Input: part model. Units: mm. Frame: model coordinates. A direction names the side the tool comes from. Round coordinates to 2 decimals unless told otherwise and drop trailing zeros. Write each loop counter-clockwise with the first axis right and the second up, starting at its lowest first coordinate (ties: lowest second). Pieces come first, ordered by that corner, then holes. Notation, with made-up numbers: (52.25, -31) -> (105.25, -31) arc R17 ccw to (105.25, -22) -> close; hole circle Ø2 at (55.25, 13.25). An arc over 180 degrees is marked (long way). Use CSV: the item, a comma, the result in double quotes.
Autodesk Inventor part; units mm, degrees
ref_plane "YZ Plane" through (0, 0, 0) normal (1, 0, 0) x (0, 1, 0)
ref_plane "XZ Plane" through (0, 0, 0) normal (0, 1, 0) x (-1, 0, 0)
ref_plane "XY Plane" through (0, 0, 0) normal (0, 0, 1) x (1, 0, 0)
sketch "Boceto1" plane through (0, 0, 0) normal (1, 0, 0) x (0, 1, 0)
  circle A0 centre (3, -6.5) radius 6.25
  line L0 (-9, 17.5) -> (-9, 20.5)
  line L1 (-9, 20.5) -> (3, 20.5)
  line L2 (3, 20.5) -> (3, 17.5)
  line L3 (3, 17.5) -> (40, 17.5)
  line L4 (40, 17.5) -> (40, -17.5)
  line L5 (40, -17.5) -> (3, -17.5)
  line L6 (3, -17.5) -> (3, -20.5)
  line L7 (3, -20.5) -> (-9, -20.5)
  line L8 (-9, -20.5) -> (-9, -17.5)
  line L9 (-9, -17.5) -> (-40, -17.5)
  line L10 (-40, -17.5) -> (-40, 17.5)
  line L11 (-40, 17.5) -> (-9, 17.5)
  point P0 (0, 0)
extrude "Extrusión1" add sketch "Boceto1" along normal blind 3
properties part number "Wheel_Support" material "MDF Tablero de fibras de densidad media"
Item 1: Line query: line 1 (Z direction, x = 1.15, y = 23); line 2 (Y direction, x = 0.35, z = -7.5). Output: solid intervals per line, ascending.
Worked answers:
line 1,"z = -17.5 to 17.5"
line 2,"y = -40 to -3.17, 9.17 to 40"
Item 2: Section query A-A on z = -1.5. Return the cut outline in (x, y), plus the area to 4 significant figures.
Worked answers:
outline,"(0, -40) -> (3, -40) -> (3, -0.75) -> (0, -0.75) -> close; (0, 6.75) -> (3, 6.75) -> (3, 40) -> (0, 40) -> close"
area,"217.5 mm²"
Item 3: Section query D-D on y = -34.5. Return the cut outline in (x, z).
Worked answers:
outline,"(0, -17.5) -> (3, -17.5) -> (3, 17.5) -> (0, 17.5) -> close"
Item 4: Set-up query: faces 1 (the face through (1, -25, 17.5)), 2 (the face through (1, -3, 20.5)), 3 (the face through (1, 22, -17.5)), 4 (the face through (1, -24, -17.5)), 5 (the face through (1, 3, 19)). Return all of +Z, -Z, +X, -X, +Y, -Y with unobstructed straight access to the full face (end or side cutting, diameter ignored); none if empty.
Worked answers:
face 1,"+Z, +X, -X, -Y"
face 2,"+Z, +X, -X, +Y, -Y"
face 3,"-Z, +X, -X, +Y"
face 4,"-Z, +X, -X, -Y"
face 5,"+Z, +X, -X, +Y"
Item 5: Section query C-C on z = -6.5. Return the cut outline in (x, y), plus the area to 4 significant figures.
Worked answers:
outline,"(0, -40) -> (3, -40) -> (3, -3.25) -> (0, -3.25) -> close; (0, 9.25) -> (3, 9.25) -> (3, 40) -> (0, 40) -> close"
area,"202.5 mm²"
Item 6: Section query B-B on x = 0.8. Return the cut outline in (y, z), plus the area to 3 significant figures.
Worked answers:
outline,"(-40, -17.5) -> (-9, -17.5) -> (-9, -20.5) -> (3, -20.5) -> (3, -17.5) -> (40, -17.5) -> (40, 17.5) -> (3, 17.5) -> (3, 20.5) -> (-9, 20.5) -> (-9, 17.5) -> (-40, 17.5) -> close; hole circle Ø12.5 at (3, -6.5)"
area,"2,750 mm²"
Item 7: Pull-direction query (Y, two-part tool) for faces 6 (the face through (1.479, 5.884, -0.955)), 7 (the face through (1, 21, 17.5)), 8 (the face through (1, -40, 0)), 9 (the face through (1, 3, -19)); classes: +Y half, -Y half, draft (parallel to the pull), parting line (faces both ways), or undercut.
Worked answers:
face 6,"undercut"
face 7,"draft"
face 8,"-Y half"
face 9,"+Y half"
Item 8: First-contact query: pin 1 Ø1.5 at (x, z) = (2, 18.5) entering from -Y; pin 2 Ø1.5 at (x, y) = (1.5, 21) entering from -Z; pin 3 Ø7.5 at (y, z) = (3, -6.5) entering from +X. Flat tips, straight axial feed; report the tip coordinate or a pass-through.
Worked answers:
pin 1,"stops at y = -9"
pin 2,"stops at z = -17.5"
pin 3,"passes through"
